Geometry check sheet. Reference: the model listing, model coordinates, mm. Face numbers are marked on the shaded views. A direction names the side the tool comes from. Give positions to 0.01 mm unless a question says otherwise; leave off trailing zeros. Write each loop counter-clockwise with the first axis right and the second up, starting at its lowest first coordinate (ties: lowest second). Pieces come first, ordered by that corner, then holes. Notation, with made-up numbers: M -34,-23.5 L -19,-23.5 A8 cw -19,-11.5 Z; hole C 87.25,-40 d4. An arc over 180 degrees is marked long. Use one line per item in the form item = value. Start each with the question number.
```python
from build123d import *

# Parameters (mm, degrees)
F1_DEPTH = 7.7
F2_R     = 1.97
F3_DEPTH = 25
F4_R     = 2.435
F5_DEPTH = 5.7
F7_DEPTH = 5


with BuildPart() as f1:
    # F0 (on Front) → F1 (new body)
    with BuildSketch(Plane.XZ):
        Polygon((-30.294312, 48.087149), (-41.234312, 48.087149), (-43.929312, 35.553619), (-27.599312, 35.553619), align=None)
    extrude(amount=F1_DEPTH)

    # F2 (on face) → F3 (cut)
    with BuildSketch(Plane(origin=(-49.295012, 0, 10.599572), x_dir=(0, -1, 0), z_dir=(-0.977654, 0, 0.210218))):
        with Locations((3.75, 34.817591)):
            Circle(F2_R)
    extrude(amount=-F3_DEPTH, mode=Mode.SUBTRACT)

    # F4 (on face) → F5 (join)
    with BuildSketch(Plane.XY.offset(48.087149)):
        with Locations((-36.07548, -3.85)):
            Circle(F4_R)
    extrude(amount=F5_DEPTH)

    # F6 (on face) → F7 (cut)
    with BuildSketch(Plane(origin=(0, 0, 35.553619), x_dir=(1, 0, 0), z_dir=(0, 0, -1))):
        Polygon((-37.525672, 2.131142), (-37.894156, 1.61), (-37.184659, 1.61), (-37.184659, 2.131142), align=None)
        Polygon((-34.179285, 2.131142), (-34.179285, 1.61), (-33.376172, 1.61), (-33.782143, 2.131142), align=None)
        Polygon((-37.184659, 6.09), (-37.894156, 6.09), (-37.525672, 5.577996), (-37.184659, 5.577996), align=None)
        Polygon((-33.376172, 6.09), (-34.179285, 6.09), (-34.179285, 5.577996), (-33.782143, 5.577996), align=None)
        Polygon((-37.894156, 6.09), (-42.319312, 6.09), (-42.319312, 1.61), (-37.894156, 1.61), (-37.525672, 2.131142), (-37.184659, 2.131142), (-37.184659, 1.61), (-34.179285, 1.61), (-34.179285, 2.131142), (-33.782143, 2.131142), (-33.376172, 1.61), (-29.209312, 1.61), (-29.209312, 6.09), (-33.376172, 6.09), (-33.782143, 5.577996), (-34.179285, 5.577996), (-34.179285, 6.09), (-37.184659, 6.09), (-37.184659, 5.577996), (-37.525672, 5.577996), align=None)
    extrude(amount=-F7_DEPTH, mode=Mode.SUBTRACT)


solid = f1.part
```
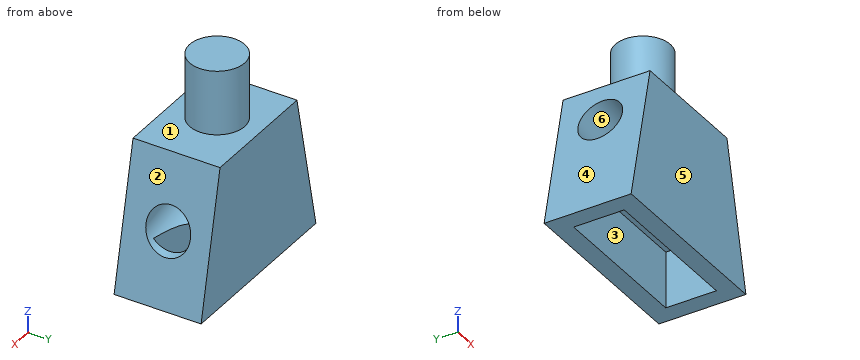
(1) Thickness scan on probe 1 along Y at (x, z) = (-38.25, 44.75); probe 2 along X at (y, z) = (-5.25, 36.5); probe 3 along Y at (x, z) = (-40.25, 43). Record the ranges inside material, lowest first. Write a range as [from, to].
(2) Sectioned sample at C-C, the plane y = -6.5. Record the boundary of the cut face in (x, z), plus the area to 3 significant figures.
(3) Sectioned sample at D-D, the plane z = 50.5. Record the boundary of the cut face in (x, y) (3 decimals), plus the area to 3 significant figures.
(4) Tool access check on the marked faces 1, 2 and 3. Record the directions out of +Z, -Z, +X, -X, +Y, -Y that give a thin tool (end or side, any length) a straight path to the whole face; none if there is none.
(5) Sectioned sample at A-A, the plane z = 39.5. Record the boundary of the cut face in (x, y), plus the area to 3 significant figures.
(6) Depth check by flat-ended pin: pin 1 (1.5 mm diameter, centred on x = -41, y = -4.5, fed in from +Z); pin 2 (3.5 mm diameter, centred on y = -4, z = 38.5, fed in from +X); pin 3 (2 mm diameter, centred on x = -34.5, y = -3, fed in from -Z). Enter the tip coordinate at first touch or a pass-through.
(7) Draft check along Z on the marked faces 4, 5 and 6. Enter one of: released by +Z, released by -Z, zero draft, split by the parting line, or undercut.
(8) Sectioned sample at B-B, the plane y = -4.25. Record the boundary of the cut face in (x, z), plus the area to 3 significant figures.
Numbers:
q1.probe_1 = [-7.7, -5.51], [-1.99, 0]
q1.probe_2 = [-43.73, -42.32], [-29.21, -27.8]
q1.probe_3 = [-7.7, -5.28], [-2.22, 0]
q2.outline = M -43.93,35.55 L -27.6,35.55 L -30.29,48.09 L -41.23,48.09 Z
q2.area = 171 mm2
q3.outline = C -36.075,-3.85 d4.87
q3.area = 18.6 mm2
q4.face_1 = +Z
q4.face_2 = +Z, +X, +Y, -Y
q4.face_3 = -Z
q5.outline = M -43.08,-7.7 L -28.45,-7.7 L -28.45,0 L -43.08,0 Z; hole M -42.32,-6.09 L -29.21,-6.09 L -29.21,-1.61 L -42.32,-1.61 Z
q5.area = 53.9 mm2
q6.pin_1 = 48.09
q6.pin_2 = -27.86
q6.pin_3 = 40.55
q7.face_4 = released by +Z
q7.face_5 = zero draft
q7.face_6 = undercut
q8.outline = M -43.93,35.55 L -42.32,35.55 L -42.32,40.55 L -32.04,40.55 L -42.38,42.78 Z; M -41.58,46.5 L -29.39,43.88 L -30.29,48.09 L -33.67,48.09 L -33.67,53.79 L -38.48,53.79 L -38.48,48.09 L -41.23,48.09 Z; M -29.21,35.55 L -27.6,35.55 L -28.51,39.79 L -29.21,39.95 Z
q8.area = 82.8 mm2
